```python
from build123d import *

# Parameters (mm, degrees)
BODY_DEPTH                             = 70
FRONTAL_M3_NUT_CUTOUTS_DEPTH           = 3
FRONTAL_M4_NUT_CUTOUT_DEPTH            = 2
MAIN_CHAMFER_SIZE                      = 5
SIDE_CHAMFER_SIZE                      = 1
WALL_CHAMFERS_SIZE                     = 10
CLEARANCE_CUTOUT_DEPTH                 = 4
M3_FULL_MIRROR_COPY_3_DEPTH            = 3
BOTTOM_BOARD_MOUNTING_HOLE_D           = 4.5
BOTTOM_BOARD_MOUNTING_HOLE_CBORE_D     = 8
BOTTOM_BOARD_MOUNTING_HOLE_CBORE_DEPTH = 4.4
BOTTOM_M4_NUT_CUTOUT_DEPTH             = 2


# Read off the part's stored shape, not the designer's step: hull_mounting_holes
with BuildPart() as part:
    # body_sketch → body (new body)
    with BuildSketch(Plane(origin=(0, 0, 0), x_dir=(0, 0, -1), z_dir=(1, 0, 0))):
        Polygon((0, 0), (0, 20), (-8, 20), (-8, 55), (-20, 55), (-20, 20), (-55, 20), (-55, 8), (-20, 8), (-20, 0), align=None)
    extrude(amount=BODY_DEPTH)

    # rod_hole_sketch_auto → rod_hole_d10 (revolve, cut)
    with BuildSketch(Plane(origin=(70, 10, 10), x_dir=(0, 0, -1), z_dir=(0, 1, 0))):
        Polygon((0, 0), (0, 70), (5.25, 70), (5.1, 69.740192379), (5.1, 0.259807621), (5.25, 0), align=None)
    revolve(axis=Axis((76.35, 10, 10), (-1, 0, 0)), mode=Mode.SUBTRACT)

    # hull_mounting_holes outline → hull_mounting_holes (revolve, cut)
    with BuildSketch(Plane(origin=(25, 45, 0), x_dir=(1, 0, 0), z_dir=(0, -1, 0))):
        Polygon((0, 8), (1.8, 8), (1.7, 8.1), (1.7, 19.9), (1.8, 20), (0, 20), align=None)
    hull_mounting_holes = revolve(axis=Axis((25, 45, 0), (0, 0, 1)), mode=Mode.SUBTRACT)

    # hull_mounting_holes 2 outline → hull_mounting_holes 2 (revolve, cut)
    with BuildSketch(Plane(origin=(10, 30, 0), x_dir=(1, 0, 0), z_dir=(0, -1, 0))):
        Polygon((0, 8), (1.8, 8), (1.7, 8.1), (1.7, 19.9), (1.8, 20), (0, 20), align=None)
    hull_mounting_holes_2 = revolve(axis=Axis((10, 30, 0), (0, 0, 1)), mode=Mode.SUBTRACT)

    # Sketch8 → board_mounting_hole (revolve, cut)
    with BuildSketch(Plane(origin=(25, 30, 8), x_dir=(0, 1, 0), z_dir=(1, 0, 0))):
        Polygon((0, 0), (0, 12), (2.275, 12), (2.25, 11.975), (2.25, 4.4), (4, 4.4), (4, 0.025), (4.025, 0), align=None)
    board_mounting_hole = revolve(axis=Axis((25, 30, 1.65), (0, 0, 1)), mode=Mode.SUBTRACT)

    # Sketch9 → frontal_m3_nut_cutouts (cut)
    with BuildSketch(Plane.XY.offset(20)):
        Polygon((25, 48.175426481), (22.25, 46.58771324), (22.25, 43.41228676), (25, 41.824573519), (27.75, 43.41228676), (27.75, 46.58771324), align=None)
        Polygon((10, 33.175426481), (7.25, 31.58771324), (7.25, 28.41228676), (10, 26.824573519), (12.75, 28.41228676), (12.75, 31.58771324), align=None)
    frontal_m3_nut_cutouts = extrude(amount=-FRONTAL_M3_NUT_CUTOUTS_DEPTH, mode=Mode.SUBTRACT)

    # Sketch10 → frontal_m4_nut_cutout (cut)
    with BuildSketch(Plane.XY.offset(20)):
        Polygon((21.5, 32.020725942), (21.5, 27.979274058), (25, 25.958548116), (28.5, 27.979274058), (28.5, 32.020725942), (25, 34.041451884), align=None)
    frontal_m4_nut_cutout = extrude(amount=-FRONTAL_M4_NUT_CUTOUT_DEPTH, mode=Mode.SUBTRACT)

    # frontal_m4_mirror: board_mounting_hole, frontal_m4_nut_cutout across plane
    add(board_mounting_hole.mirror(Plane.ZY.offset(-35)), mode=Mode.SUBTRACT)
    add(frontal_m4_nut_cutout.mirror(Plane.ZY.offset(-35)), mode=Mode.SUBTRACT)

    # main_chamfer
    main_chamfer_edges = [part.edges().sort_by_distance(p)[0] for p in [
        (35, 0, 0),
    ]]
    chamfer(main_chamfer_edges, length=MAIN_CHAMFER_SIZE)

    # side_chamfer
    side_chamfer_edges = [part.edges().sort_by_distance(p)[0] for p in [
        (0, 4, 20),
        (70, 20, 4),
        (0, 20, 4),
        (0, 0, 12.5),
        (0, 12.5, 0),
        (70, 12.5, 0),
        (0, 2.5, 2.5),
        (70, 2.5, 2.5),
        (35, 0, 20),
        (35, 20, 0),
        (70, 4, 20),
        (70, 0, 12.5),
    ]]
    chamfer(side_chamfer_edges, length=SIDE_CHAMFER_SIZE)

    # wall_chamfers
    wall_chamfers_edges = [part.edges().sort_by_distance(p)[0] for p in [
        (0, 14, 55),
        (0, 55, 14),
        (70, 55, 14),
        (70, 14, 55),
    ]]
    chamfer(wall_chamfers_edges, length=WALL_CHAMFERS_SIZE)

    # Sketch11 → clearance_cutout (cut)
    with BuildSketch(Plane.XY.offset(20)):
        Polygon((0, 20), (5, 20), (5, 40), (15, 50), (55, 50), (65, 40), (65, 20), (70, 20), (70, 45), (60, 55), (10, 55), (0, 45), align=None)
    extrude(amount=-CLEARANCE_CUTOUT_DEPTH, mode=Mode.SUBTRACT)

    # bottom_m3_mirror: hull_mounting_holes, hull_mounting_holes 2, frontal_m3_nut_cutouts across plane
    add(hull_mounting_holes.mirror(Plane(origin=(0, 0, 0), x_dir=(0, 0.7071067811865476, 0.7071067811865475), z_dir=(0, 0.7071067811865475, -0.7071067811865476))), mode=Mode.SUBTRACT)
    add(hull_mounting_holes_2.mirror(Plane(origin=(0, 0, 0), x_dir=(0, 0.7071067811865476, 0.7071067811865475), z_dir=(0, 0.7071067811865475, -0.7071067811865476))), mode=Mode.SUBTRACT)
    add(frontal_m3_nut_cutouts.mirror(Plane(origin=(0, 0, 0), x_dir=(0, 0.7071067811865476, 0.7071067811865475), z_dir=(0, 0.7071067811865475, -0.7071067811865476))), mode=Mode.SUBTRACT)

    # m3_full_mirror: hull_mounting_holes, hull_mounting_holes 2, frontal_m3_nut_cutouts across plane
    add(hull_mounting_holes.mirror(Plane.ZY.offset(-35)), mode=Mode.SUBTRACT)
    add(hull_mounting_holes_2.mirror(Plane.ZY.offset(-35)), mode=Mode.SUBTRACT)
    add(frontal_m3_nut_cutouts.mirror(Plane.ZY.offset(-35)), mode=Mode.SUBTRACT)

    # m3_full_mirror copy 1 sketch → m3_full_mirror copy 1 (revolve, cut)
    with BuildSketch(Plane(origin=(45, 0, 45), x_dir=(-1, 0, 0), z_dir=(0, 0, -1))):
        Polygon((0, 8), (1.8, 8), (1.7, 8.1), (1.7, 19.9), (1.8, 20), (0, 20), align=None)
    revolve(axis=Axis((45, 0, 45), (0, 1, 0)), mode=Mode.SUBTRACT)

    # m3_full_mirror copy 2 sketch → m3_full_mirror copy 2 (revolve, cut)
    with BuildSketch(Plane(origin=(60, 0, 30), x_dir=(-1, 0, 0), z_dir=(0, 0, -1))):
        Polygon((0, 8), (1.8, 8), (1.7, 8.1), (1.7, 19.9), (1.8, 20), (0, 20), align=None)
    revolve(axis=Axis((60, 0, 30), (0, 1, 0)), mode=Mode.SUBTRACT)

    # m3_full_mirror copy 3 sketch → m3_full_mirror copy 3 (cut)
    with BuildSketch(Plane(origin=(70, 20, 0), x_dir=(-1, 0, 0), z_dir=(0, 1, 0))):
        Polygon((25, 48.175426481), (22.25, 46.58771324), (22.25, 43.41228676), (25, 41.824573519), (27.75, 43.41228676), (27.75, 46.58771324), align=None)
        Polygon((10, 33.175426481), (7.25, 31.58771324), (7.25, 28.41228676), (10, 26.824573519), (12.75, 28.41228676), (12.75, 31.58771324), align=None)
    extrude(amount=-M3_FULL_MIRROR_COPY_3_DEPTH, mode=Mode.SUBTRACT)

    # m3_full_mirror copy 4 sketch → m3_full_mirror copy 4 (revolve, cut)
    with BuildSketch(Plane(origin=(60, 30, 0), x_dir=(-1, 0, 0), z_dir=(0, -1, 0))):
        Polygon((0, -8), (1.8, -8), (1.7, -8.1), (1.7, -19.9), (1.8, -20), (0, -20), align=None)
    revolve(axis=Axis((60, 30, 0), (0, 0, -1)), mode=Mode.SUBTRACT)

    # bottom_board_mounting_hole (through all)
    with Locations(Plane.XZ.offset(-8)):
        with Locations((10, 45)):
            bottom_board_mounting_hole = CounterBoreHole(BOTTOM_BOARD_MOUNTING_HOLE_D / 2, BOTTOM_BOARD_MOUNTING_HOLE_CBORE_D / 2, BOTTOM_BOARD_MOUNTING_HOLE_CBORE_DEPTH)

    # Sketch15 → bottom_m4_nut_cutout (cut)
    with BuildSketch(Plane(origin=(0, 20, 0), x_dir=(1, 0, 0), z_dir=(0, 1, 0))):
        Polygon((10, -40.958548116), (6.5, -42.979274058), (6.5, -47.020725942), (10, -49.041451884), (13.5, -47.020725942), (13.5, -42.979274058), align=None)
    bottom_m4_nut_cutout = extrude(amount=-BOTTOM_M4_NUT_CUTOUT_DEPTH, mode=Mode.SUBTRACT)

    # bottom_m4_mirror: bottom_board_mounting_hole, bottom_m4_nut_cutout across plane
    add(bottom_board_mounting_hole.mirror(Plane.ZY.offset(-35)), mode=Mode.SUBTRACT)
    add(bottom_m4_nut_cutout.mirror(Plane.ZY.offset(-35)), mode=Mode.SUBTRACT)


solid = part.part
```
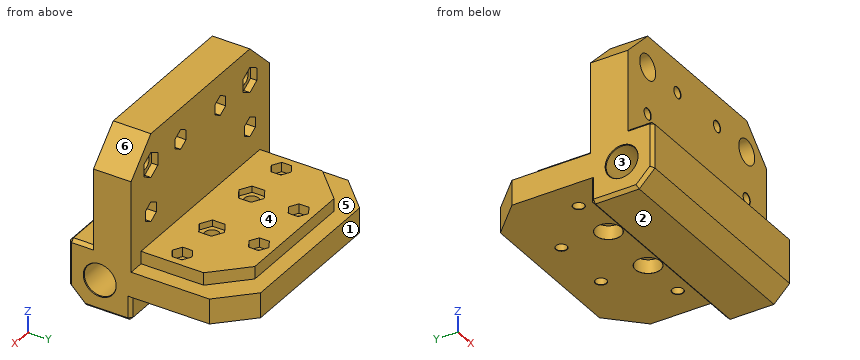
Geometry check sheet. Reference: the model listing, model coordinates, mm. Face numbers are marked on the shaded views. A direction names the side the tool comes from. Coordinates: 2 decimals unless noted, no trailing zeros. Write each loop counter-clockwise with the first axis right and the second up, starting at its lowest first coordinate (ties: lowest second). Pieces come first, ordered by that corner, then holes. Notation, with made-up numbers: M 18,71 L 24,71 A19 ccw 24,92 Z; hole C -40,26.25 d8. An arc over 180 degrees is marked long. Use one line per item in the form item = value. Start each with the question number.
1) Section check A-A on z = 30. Enter the section's corners in (x, y).
2) Thickness scan on probe 1 along Z at (x, y) = (27, 10); probe 2 along X at (y, z) = (12.5, 43); probe 3 along Z at (x, y) = (55, 51). Record the ranges inside material, lowest first. Write a range as from..to.
3) Release check for a two-part mould opening along Y. For the marked faces 1, 2 and 3 record: pulls with the +Y half, pulls with the -Y half, needs draft (parallel to the pull), parting line crosses it, or undercut.
4) Section check B-B on y = 22.5. Enter the section's corners in (x, z), and give its area (3 significant figures).
5) Go/stop test with flat-tipped pins: pin 1 Ø2 at (x, z) = (47, 32) entering from -Y; pin 2 Ø1 at (y, z) = (11, 47.5) entering from -X; pin 3 Ø8 at (x, y) = (47.5, 25.5) entering from -Z. Record where each tip stops, or that it passes through.
6) Set-up check for the marked faces 4, 5 and 6: record each of +Z, -Z, +X, -X, +Y, -Y from which the full face is reachable in a straight line by a thin tool's end or side.
7) Section check C-C on y = 30. State how many separate pieces and enclosed holes the cut face has, and give its area (3 significant figures).
Responses:
q1.outline = M 0,8 L 8.2,8 L 8.3,8.1 L 8.3,17 L 7.25,17 L 7.25,20 L 0,20 Z; M 11.7,8.1 L 11.8,8 L 58.2,8 L 58.3,8.1 L 58.3,17 L 57.25,17 L 57.25,20 L 12.75,20 L 12.75,17 L 11.7,17 Z; M 61.7,8.1 L 61.8,8 L 70,8 L 70,20 L 62.75,20 L 62.75,17 L 61.7,17 Z
q2.probe_1 = 0..4.9, 15.1..55
q2.probe_2 = 0..8.97, 11.03..58.97, 61.03..70
q2.probe_3 = 8..16
q3.face_1 = pulls with the +Y half
q3.face_2 = needs draft
q3.face_3 = undercut
q4.outline = M 0,8 L 70,8 L 70,16 L 65,16 L 65,20 L 5,20 L 5,16 L 0,16 Z
q4.area = 800 mm2
q5.pin_1 = 8
q5.pin_2 = 2
q5.pin_3 = 8
q6.face_4 = +Z, +X, -X, +Y
q6.face_5 = +Z, +Y
q6.face_6 = +Z, +X, +Y, -Y
q7.separate_pieces = 5
q7.enclosed_holes = 0
q7.area = 557 mm2
